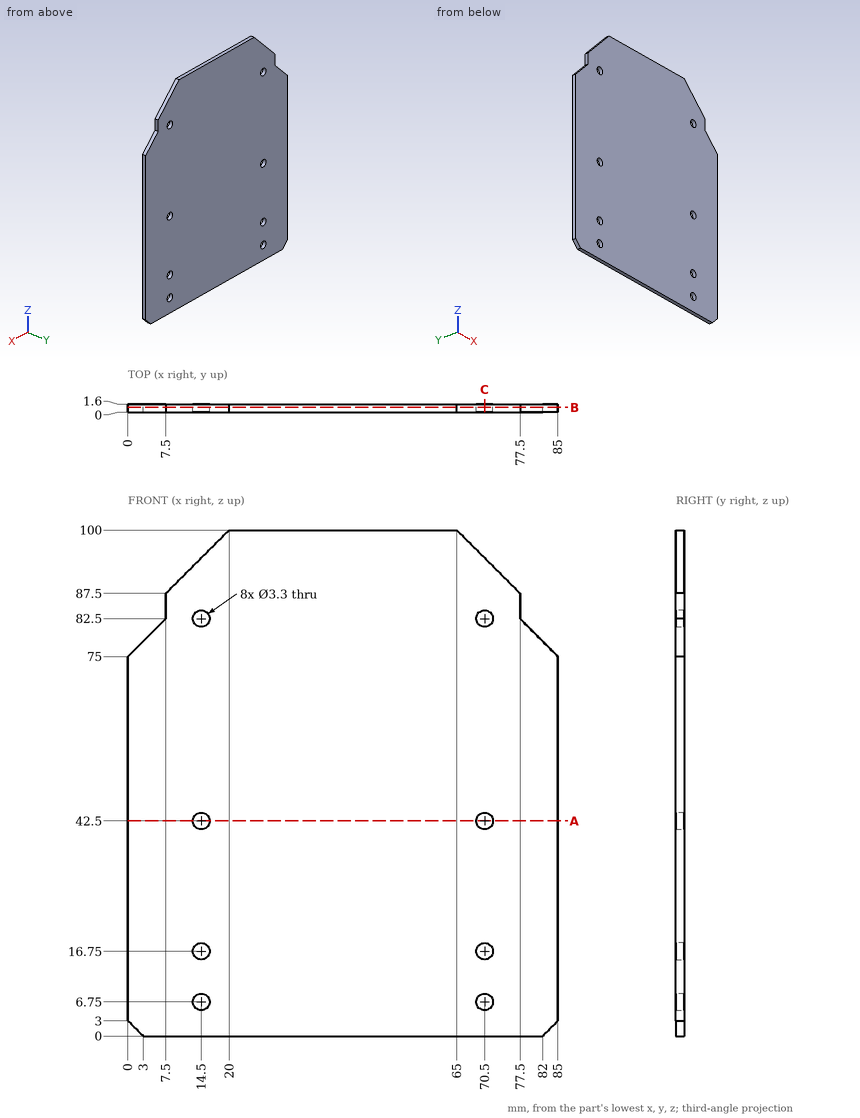
Could you check a few things on this drawing? It's one solid part, dimensions in mm from its lowest x, y, z. Coordinates: 2 decimals unless noted, no trailing zeros. Write each loop counter-clockwise with the first axis right and the second up, starting at its lowest first coordinate (ties: lowest second). Pieces come first, ordered by that corner, then holes. Notation, with made-up numbers: (41.25, 57.25) - (49.25, 57.25) arc R20 cw to (49.25, 96.25) - close; hole circle Ø2 at (-40, -19.75). An arc over 180 degrees is marked (long way). Use one line per item in the form item = value.
1) I'm going to push flat-ended pins straight in: P1, Ø2.5, axis at x = 70.5, z = 82.5, coming from the +Y side; P2, Ø0.8, axis at y = 0.5, z = 85, coming from the -X side. Where does each tip first touch, or does it pass through?
Solved:
P1 = through
P2 = 7.5
2) Suppose I cut it at B-B, the plane y = 0.95. Give the number of separate pieces and of enclosed holes in the cut face, plus the area to 3 significant figures.
Solved:
separate_pieces = 1
enclosed_holes = 8
area = 7,950 mm2
3) I need wall thicknesses on line 1 (X direction, y = 0.45, z = 6.75); line 2 (X direction, y = 0.95, z = 82.5); line 3 (Z direction, x = 70.5, y = 1). Which ranges of each line are inside material? Lowest first, please.
Solved:
line_1 = 0 to 12.85, 16.15 to 68.85, 72.15 to 85
line_2 = 7.5 to 12.85, 16.15 to 68.85, 72.15 to 77.5
line_3 = 0 to 5.1, 8.4 to 15.1, 18.4 to 40.85, 44.15 to 80.85, 84.15 to 94.5
4) Suppose I cut it at C-C, the plane x = 70.5. Write out the boundary of the cut face in (y, z).
Solved:
outline = (0, 0) - (1.6, 0) - (1.6, 5.1) - (0, 5.1) - close; (0, 8.4) - (1.6, 8.4) - (1.6, 15.1) - (0, 15.1) - close; (0, 18.4) - (1.6, 18.4) - (1.6, 40.85) - (0, 40.85) - close; (0, 44.15) - (1.6, 44.15) - (1.6, 80.85) - (0, 80.85) - close; (0, 84.15) - (1.6, 84.15) - (1.6, 94.5) - (0, 94.5) - close
5) Suppose I cut it at A-A, the plane z = 42.5. Write out the boundary of the cut face in (x, y).
Solved:
outline = (0, 0) - (12.85, 0) - (12.85, 1.6) - (0, 1.6) - close; (16.15, 0) - (68.85, 0) - (68.85, 1.6) - (16.15, 1.6) - close; (72.15, 0) - (85, 0) - (85, 1.6) - (72.15, 1.6) - close
